Model file for the job. Use its own axes, mm. Give positions to 0.01 mm unless a question says otherwise; leave off trailing zeros. Loops run counter-clockwise (first coordinate to the right, second up) from the corner with the lowest first, then second, coordinate; pieces in that order, holes last. Notation, with made-up numbers: (19.25, 7) -> (33.25, 7) arc R31 ccw to (33.25, 43) -> close; hole circle Ø6 at (32.5, 31.25). An arc over 180 degrees is marked (long way). Use CSV: the item, a comma, the result in double quotes. Start each with the question number.
(1) Drill centre lines: probe 1 along Z at (x, y) = (22.5, -16.25); probe 2 along Z at (x, y) = (31.5, -4.25); probe 3 along X at (y, z) = (-5.75, -32.5). Where is each one in solid material? Low to high.
(2) Cut at B-B on x = -23. Write the cut outline in (y, z).
(3) Cut at C-C on z = -31. Write the cut outline in (x, y).
(4) Flat gauge pins, fed straight in: pin 1 (10 mm diameter, centred on x = -45, y = -15, fed in from +Z); pin 2 (2 mm diameter, centred on x = 28, y = -14, fed in from +Z). Where does each tip first touch, or does it go through?
(5) Cut at A-A on y = -9. Write the cut outline in (x, z), then the cut area to 3 significant figures.
from build123d import *

# Parameters (mm, degrees)
F0_W     = 127
F0_H     = 76.2
F1_DEPTH = 19.05
F2_SIZE  = 20.32
F3_SIZE  = 7.62


with BuildPart() as f1:
    # F0 (on Front) → F1 (new body)
    with BuildSketch(Plane.XZ):
        with Locations((-18.789873, -52.389765)):
            Rectangle(F0_W, F0_H)
    extrude(amount=F1_DEPTH)

    # F2
    f2_edges = [f1.edges().sort_by_distance(p)[0] for p in [
        (44.710127, -9.525, -14.289765),
        (-82.289873, -9.525, -14.289765),
    ]]
    chamfer(f2_edges, length=F2_SIZE)

    # F3
    f3_edges = [f1.edges().sort_by_distance(p)[0] for p in [
        (-18.789873, -19.05, -14.289765),
        (-18.789873, 0, -14.289765),
    ]]
    chamfer(f3_edges, length=F3_SIZE)


solid = f1.part
Check result:
1,probe 1,"-90.49 to -19.11"
1,probe 2,"-90.49 to -21.4"
1,probe 3,"-80.18 to 42.6"
2,outline,"(-19.05, -90.49) -> (0, -90.49) -> (0, -21.91) -> (-7.62, -14.29) -> (-11.43, -14.29) -> (-19.05, -21.91) -> close"
3,outline,"(-78.68, -19.05) -> (41.1, -19.05) -> (41.1, 0) -> (-78.68, 0) -> close"
4,pin 1,"z = -14.29"
4,pin 2,"z = -16.9"
5,outline,"(-82.29, -90.49) -> (44.71, -90.49) -> (44.71, -34.61) -> (24.39, -14.29) -> (-61.97, -14.29) -> (-82.29, -34.61) -> close"
5,area,"9,260 mm²"
